Geometry: final body of the model. Coordinates: model frame, mm. Face numbers are marked on the shaded views. A direction names the side the tool comes from. Give positions to 0.01 mm unless a question says otherwise; leave off trailing zeros. Write each loop counter-clockwise with the first axis right and the second up, starting at its lowest first coordinate (ties: lowest second). Pieces come first, ordered by that corner, then holes.
```python
from build123d import *

# Parameters (mm, degrees)
BOSS_EXTRUDE1_DEPTH = 10
SKETCH2_R           = 2
CUT_EXTRUDE2_DEPTH  = 10
SKETCH3_W           = 10
SKETCH3_H           = 10
CUT_EXTRUDE3_DEPTH  = 10


with BuildPart() as part:
    # Sketch1 → Boss-Extrude1 (new body)
    with BuildSketch(Plane.XY):
        Polygon((-57.4285121, -21.353337692), (-37.4285121, -21.353337692), (-35.4285121, -21.353337692), (-35.4285121, 6.646662308), (24.5714879, 6.646662308), (24.5714879, -21.353337692), (26.5714879, -21.353337692), (46.5714879, -21.353337692), (46.5714879, -19.353337692), (26.5714879, -19.353337692), (26.5714879, 8.646662308), (24.5714879, 8.646662308), (-35.4285121, 8.646662308), (-37.4285121, 8.646662308), (-37.4285121, -19.353337692), (-57.4285121, -19.353337692), align=None)
    extrude(amount=BOSS_EXTRUDE1_DEPTH)

    # Sketch2 → Cut-Extrude2 (cut)
    with BuildSketch(Plane(origin=(0, -19.353337692, 0), x_dir=(1, 0, 0), z_dir=(0, 1, 0))):
        with Locations((-42.4285121, -5)):
            Circle(SKETCH2_R)
        with Locations((31.5714879, -5)):
            Circle(SKETCH2_R)
    extrude(amount=-CUT_EXTRUDE2_DEPTH, mode=Mode.SUBTRACT)

    # Sketch3 → Cut-Extrude3 (cut)
    with BuildSketch(Plane(origin=(0, -19.353337692, 0), x_dir=(1, 0, 0), z_dir=(0, 1, 0))):
        with Locations((-52.4285121, -5)):
            Rectangle(SKETCH3_W, SKETCH3_H)
        with Locations((41.5714879, -5)):
            Rectangle(SKETCH3_W, SKETCH3_H)
    extrude(amount=-CUT_EXTRUDE3_DEPTH, mode=Mode.SUBTRACT)


solid = part.part
```
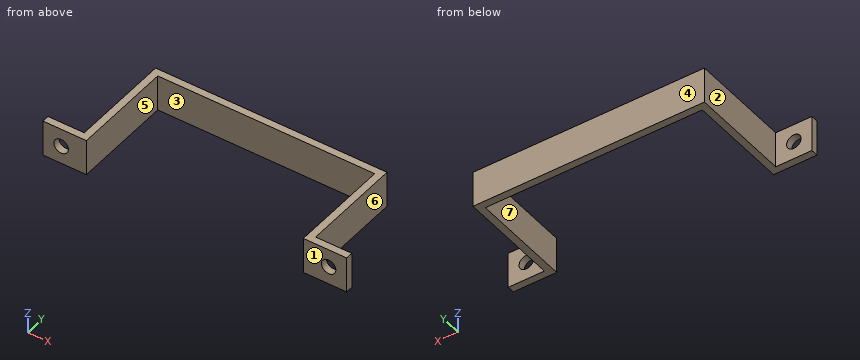
Item 1: Section A-A, the plane y = -1.5. Return the cut outline in (x, z).
Found:
outline: (-37.43, 0) - (-35.43, 0) - (-35.43, 10) - (-37.43, 10) - close; (24.57, 0) - (26.57, 0) - (26.57, 10) - (24.57, 10) - close
Item 2: Reachability of the marked faces 1, 2 and 3 from +Z, -Z, +X, -X, +Y, -Y: full face, straight path, thin tool, end or side. Return the list, or none.
Found:
face 1: +Z, -Z, +X, -X, -Y
face 2: +Z, -Z, -X, +Y
face 3: +Z, -Z, -Y
Item 3: Line query: L1, parallel to X at y = -20.2, z = 5; L2, parallel to X at y = -20, z = 1.5; L3, parallel to X at y = 4.5, z = 0.75. Output: solid intervals per line, ascending.
Found:
L1: x = -47.43 to -44.43, -40.43 to -35.43, 24.57 to 29.57, 33.57 to 36.57
L2: x = -47.43 to -35.43, 24.57 to 36.57
L3: x = -37.43 to -35.43, 24.57 to 26.57
Item 4: Pin query (flat end, axial travel): pin 1 Ø4.5 at (x, z) = (-42.43, 5) entering from +Y; pin 2 Ø1 at (x, z) = (-21.5, 2.5) entering from -Y; pin 3 Ø3 at (y, z) = (-10, 4) entering from +X. Return the tip coordinate at first contact, or that it passes through.
Found:
pin 1: stops at y = -19.35
pin 2: stops at y = 6.65
pin 3: stops at x = 26.57
Item 5: Pull-direction query (X, two-part tool) for the marked faces 4, 5, 6 and 7; classes: +X half, -X half, draft (parallel to the pull), parting line (faces both ways), or undercut.
Found:
face 4: draft
face 5: undercut
face 6: +X half
face 7: undercut
Item 6: Section B-B, the plane z = 5. Return the cut outline in (x, y).
Found:
outline: (-47.43, -21.35) - (-44.43, -21.35) - (-44.43, -19.35) - (-47.43, -19.35) - close; (-40.43, -21.35) - (-35.43, -21.35) - (-35.43, 6.65) - (24.57, 6.65) - (24.57, -21.35) - (29.57, -21.35) - (29.57, -19.35) - (26.57, -19.35) - (26.57, 8.65) - (-37.43, 8.65) - (-37.43, -19.35) - (-40.43, -19.35) - close; (33.57, -21.35) - (36.57, -21.35) - (36.57, -19.35) - (33.57, -19.35) - close
Item 7: Section C-C, the plane z = 1. Return the cut outline in (x, y).
Found:
outline: (-47.43, -21.35) - (-35.43, -21.35) - (-35.43, 6.65) - (24.57, 6.65) - (24.57, -21.35) - (36.57, -21.35) - (36.57, -19.35) - (26.57, -19.35) - (26.57, 8.65) - (-37.43, 8.65) - (-37.43, -19.35) - (-47.43, -19.35) - close
Item 8: Section D-D, the plane x = -29. Return the cut outline in (y, z), plus the area to 3 significant figures.
Found:
outline: (6.65, 0) - (8.65, 0) - (8.65, 10) - (6.65, 10) - close
area: 20.0 mm2
